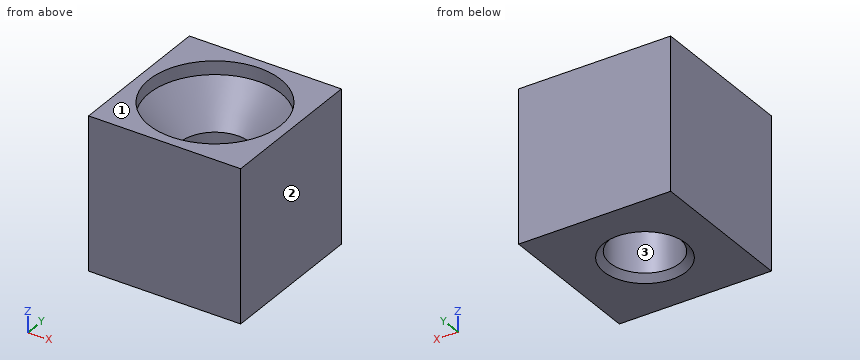
from build123d import *

# Parameters (mm, degrees)
SKETCH1_W           = 12
SKETCH1_H           = 12
SKETCH1_R           = 2.75
BOSS_EXTRUDE1_DEPTH = 12
SKETCH2_R           = 5.2
CUT_EXTRUDE1_DEPTH  = 1
CHAMFER1_SIZE       = 3
CHAMFER1_SIZE_2     = 2.5
CHAMFER2_SIZE       = 0.5


with BuildPart() as part:
    # Sketch1 → Boss-Extrude1 (new body)
    with BuildSketch(Plane.XY):
        Rectangle(SKETCH1_W, SKETCH1_H)
        Circle(SKETCH1_R, mode=Mode.SUBTRACT)
    extrude(amount=BOSS_EXTRUDE1_DEPTH)

    # Sketch2 → Cut-Extrude1 (cut)
    with BuildSketch(Plane.XY.offset(12)):
        Circle(SKETCH2_R)
    extrude(amount=-CUT_EXTRUDE1_DEPTH, mode=Mode.SUBTRACT)

    # Chamfer1
    # the kernel refuses this chamfer: 3, 2.5 mm, written as the material it takes off along each edge
    with BuildSketch(Plane(origin=(0, 0, 11), x_dir=(1, 0, 0), z_dir=(0, 1, 0))) as chamfer1_piece_1_section:
        Polygon((2.75, CHAMFER1_SIZE), (2.75 + CHAMFER1_SIZE_2, 0), (2.75, 0), align=None)
    chamfer1_piece_1 = revolve(axis=Axis((0, 0, 11), (0, 0, -1)), mode=Mode.PRIVATE)
    chamfer1_piece_1 = chamfer1_piece_1 & Plane(origin=(0, 0, 9.452892591), x_dir=(1, 0, 0), z_dir=(0, 0, 1)) * Cylinder(5.2, 21, mode=Mode.PRIVATE)
    add(chamfer1_piece_1, mode=Mode.SUBTRACT)

    # Chamfer2
    chamfer2_edges = [part.edges().sort_by_distance(p)[0] for p in [
        (-2.75, 0, 0),
    ]]
    chamfer(chamfer2_edges, length=CHAMFER2_SIZE)


solid = part.part
Read the model definition and answer for the solid it produces. Units are mm, in the model's axes. Face numbers are marked on the shaded views. Give positions to 0.01 mm unless a question says otherwise; leave off trailing zeros. Write each loop counter-clockwise with the first axis right and the second up, starting at its lowest first coordinate (ties: lowest second). Pieces come first, ordered by that corner, then holes. Notation, with made-up numbers: (78, 41) - (94, 41) arc R14 cw to (94, 52) - close; hole circle Ø5 at (-2, 50). An arc over 180 degrees is marked (long way). Return JSON: item names as keys, results as strings.
Q1. A cutting plane is placed at C-C, the plane z = 4.75. Determine the outline of the cut face in (x, y), and give its area (3 significant figures).
Reply:
{"outline": "(-6, -6) - (6, -6) - (6, 6) - (-6, 6) - close; hole circle Ø5.5 at (0, 0)", "area": "120 mm²"}
Q2. A cutting plane is placed at A-A, the plane x = 0. Determine the outline of the cut face in (y, z).
Reply:
{"outline": "(-6, 0) - (-3.25, 0) - (-2.75, 0.5) - (-2.75, 8) - (-5.2, 10.94) - (-5.2, 12) - (-6, 12) - close; (2.75, 0.5) - (3.25, 0) - (6, 0) - (6, 12) - (5.2, 12) - (5.2, 10.94) - (2.75, 8) - close"}
Q3. For a pull along X with two mould halves and no side action, classify the marked faces 1, 2 and 3 as released by +X, released by -X, zero draft, split by the parting line, or undercut.
Reply:
{"face 1": "zero draft", "face 2": "released by +X", "face 3": "undercut"}
Q4. Consider line 1 along X through (y, z) = (0, 3.5); line 2 along Y through (x, z) = (0, 11.3). Determine where each line is inside the solid, lowest interval first. Write a range as [from, to].
Reply:
{"line 1": "[-6, -2.75], [2.75, 6]", "line 2": "[-6, -5.2], [5.2, 6]"}
